```python
from build123d import *

# Parameters (mm, degrees)
F1_DEPTH = 24
F3_DEPTH = 50
F4_R     = 5


with BuildPart() as f1:
    # F0 (on Top) → F1 (new body)
    with BuildSketch(Plane.XY):
        with BuildLine():
            Line((-10, 0), (-10, 31.5))
            Line((-10, 31.5), (-110, 31.5))
            Line((-110, 31.5), (-110, 0))
            Line((-110, 0), (13.9543726236, -30.5828956689))
            ThreePointArc((13.9543726236, -30.5828956689), (-3.2985610707, -19.4237321033), (-10, 0))
        make_face()
        with BuildLine():
            Line((53, 31.5), (-10, 31.5))
            Line((-10, 31.5), (-10, 0))
            ThreePointArc((-10, 0), (-3.2985610707, -19.4237321033), (13.9543726236, -30.5828956689))
            ThreePointArc((13.9543726236, -30.5828956689), (40.9237321033, -24.7985610707), (53, 0))
            Line((53, 0), (53, 31.5))
        make_face()
        with BuildLine():
            ThreePointArc((43, 0), (21.5, -21.5), (0, 0))
            Line((0, 0), (0, 21.5))
            Line((0, 21.5), (43, 21.5))
            Line((43, 21.5), (43, 0))
        make_face(mode=Mode.SUBTRACT)
    extrude(amount=F1_DEPTH)

    # F2 (on face) → F3 (join)
    with BuildSketch(Plane.XY.offset(24)):
        Polygon((-80, -7.4018112524), (-80, 31.5), (-110, 31.5), (-110, 0), align=None)
    extrude(amount=F3_DEPTH)

    # F4
    f4_edges = [f1.edges().sort_by_distance(p)[0] for p in [
        (-110, 31.5, 37),
        (-110, 15.75, 74),
        (-110, 0, 37),
        (-110, 15.75, 0),
        (-80, 12.049094, 74),
        (-95, 31.5, 74),
        (-95, -3.700906, 74),
        (-80, -7.401811, 49),
        (-80, 31.5, 49),
        (-80, 12.049094, 24),
        (-13.5, 31.5, 24),
        (53, 15.75, 24),
        (40.923732, -24.798561, 24),
        (-33.022814, -18.992353, 24),
    ]]
    fillet(f4_edges, radius=F4_R)


solid = f1.part
```
Geometry: final body of the model. Coordinates: model frame, mm. A direction names the side the tool comes from. Coordinates: 2 decimals unless noted, no trailing zeros. Loops run counter-clockwise (first coordinate to the right, second up) from the corner with the lowest first, then second, coordinate; pieces in that order, holes last. Notation, with made-up numbers: (69, 39) -> (128, 39) arc R15 cw to (128, 61) -> close; hole circle Ø9 at (-17, 38). An arc over 180 degrees is marked (long way). Use a Markdown table: item, result. Add a question column.
(1) Access query for faces 5 (the flat face through (43, 11, 12)), 6 (the cylindrical face through (-81.43, 30, 49.28)), 7 (the cylindrical face through (-95.698, -1.98, 72.574)). Directions: +Z, -Z, +X, -X, +Y, -Y. A direction counts if a zero-diameter tool reaches every point of the face in a straight line with its end or side. Return the directions, or none.
(2) Line query: line 1 along X through (y, z) = (10.5, 13); line 2 along X through (y, z) = (19, 20.5); line 3 along X through (y, z) = (21.5, 33). Output: solid intervals per line, ascending.
(3) Section query A-A, the plane y = 17. Return loops of the section in (x, z), plus the area to 3 significant figures.
(4) Pin query (flat end, axial travel): pin 1 Ø10 at (y, z) = (18.5, 30.5) entering from +X; pin 2 Ø14 at (y, z) = (13, 40.5) entering from +X; pin 3 Ø12 at (x, y) = (-18, 15.5) entering from +Z. Return the tip coordinate at first contact, or that it passes through.
(5) Mould query, pull axis Y, two halves, no side actions, for faces 1 (the flat face through (0, 11, 12)), 2 (the cylindrical face through (-108.965, 0.87, 34.091)), 3 (the cylindrical face through (21.973, -21.495, 11.832)), 4 (the cylindrical face through (-11.9, 30, 22.57)). Classes: pulls with the +Y half, pulls with the -Y half, needs draft (parallel to the pull), parting line crosses it, or undercut.
(6) Section query C-C, the plane z = 47. Return loops of the section in (x, y), plus the area to 3 significant figures.
(7) Section query B-B, the plane z = 16. Return loops of the section in (x, y).
Answer:
| question | item | result |
|---|---|---|
| 1 | face 5 | +Z, -Z |
| 1 | face 6 | +Z, +X, +Y |
| 1 | face 7 | +Z, -X, -Y |
| 2 | line 1 | x = -110 to 0, 43 to 53 |
| 2 | line 2 | x = -110 to 0, 43 to 52.77 |
| 2 | line 3 | x = -110 to -80 |
| 3 | outline | (-110, 5) arc R5 ccw to (-105, 0) -> (0, 0) -> (0, 24) -> (-75, 24) arc R5 cw to (-80, 29) -> (-80, 69) arc R5 ccw to (-85, 74) -> (-105, 74) arc R5 ccw to (-110, 69) -> close; (43, 0) -> (53, 0) -> (53, 19) arc R5 ccw to (48, 24) -> (43, 24) -> close |
| 3 | area | 4,360 mm^2 |
| 4 | pin 1 | stops at x = -78.57 |
| 4 | pin 2 | stops at x = -80 |
| 4 | pin 3 | stops at z = 24 |
| 5 | face 1 | undercut |
| 5 | face 2 | pulls with the -Y half |
| 5 | face 3 | undercut |
| 5 | face 4 | pulls with the +Y half |
| 6 | outline | (-110, 3.92) arc R5 ccw to (-106.2, -0.94) -> (-86.2, -5.87) arc R5 ccw to (-80, -1.02) -> (-80, 26.5) arc R5 ccw to (-85, 31.5) -> (-105, 31.5) arc R5 ccw to (-110, 26.5) -> close |
| 6 | area | 1,030 mm^2 |
| 7 | outline | (-110, 3.92) arc R5 ccw to (-106.2, -0.94) -> (13.95, -30.58) arc R31.5 ccw to (53, 0) -> (53, 31.5) -> (-105, 31.5) arc R5 ccw to (-110, 26.5) -> close; hole (0, 0) arc R21.5 ccw to (43, 0) -> (43, 21.5) -> (0, 21.5) -> close |
